```python
from build123d import *

# Parameters (mm, degrees)
F0_R     = 15
F0_R_2   = 9.5
F0_R_3   = 4.5
F0_R_4   = 2.55
F1_DEPTH = 15
F3_DEPTH = 3
F4_DEPTH = 10
F5_DEPTH = 5


with BuildPart() as f1:
    # F0 (on Top) → F1 (new body)
    with BuildSketch(Plane.XY):
        Circle(F0_R)
        Circle(F0_R_2, mode=Mode.SUBTRACT)
        Circle(F0_R_2)
        Circle(F0_R_3, mode=Mode.SUBTRACT)
        Circle(F0_R_3)
        Circle(F0_R_4, mode=Mode.SUBTRACT)
    extrude(amount=F1_DEPTH)

    # F2 (on face) → F3 (cut)
    with BuildSketch(Plane.XY.offset(15)):
        Polygon((2.4248711306, -4.2), (4.8497422612, 0), (2.4248711306, 4.2), (-2.4248711306, 4.2), (-4.8497422612, 0), (-2.4248711306, -4.2), align=None)
    extrude(amount=-F3_DEPTH, mode=Mode.SUBTRACT)

    # F0 (on Top) → F4 (cut)
    with BuildSketch(Plane.XY):
        Circle(F0_R_3)
        Circle(F0_R_4, mode=Mode.SUBTRACT)
    extrude(amount=F4_DEPTH, mode=Mode.SUBTRACT)

    # F0 (on Top) → F5 (join)
    with BuildSketch(Plane.XY):
        Circle(F0_R)
        Circle(F0_R_2, mode=Mode.SUBTRACT)
    extrude(amount=-F5_DEPTH)


solid = f1.part
```
Input: part model. Units: mm. Frame: model coordinates. A direction names the side the tool comes from. Give positions to 0.01 mm unless a question says otherwise; leave off trailing zeros. Order: outer loops, then holes, each group sorted by start corner. A loop starts at its lowest first (then second) coordinate and runs counter-clockwise, first axis right, second up. Notation, with made-up numbers: M -34,82.5 L -6,82.5 A29 cw -6,120.5 Z; hole C 87,-21 d8. An arc over 180 degrees is marked long. Return JSON: item names as keys, results as strings.
1) Section query A-A on x = 0. Output: boundary loops of the cut face in (y, z).
Taken from the geometry:
{"outline": "M -15,-5 L -9.5,-5 L -9.5,0 L -4.5,0 L -4.5,10 L -2.55,10 L -2.55,12 L -4.2,12 L -4.2,15 L -15,15 Z; M 2.55,10 L 4.5,10 L 4.5,0 L 9.5,0 L 9.5,-5 L 15,-5 L 15,15 L 4.2,15 L 4.2,12 L 2.55,12 Z"}
2) Section query B-B on z = 9. Output: boundary loops of the cut face in (x, y).
Taken from the geometry:
{"outline": "C 0,0 d30; hole C 0,0 d9"}
3) Line query: L1, parallel to Y at x = 0, z = 5.5; L2, parallel to Z at x = 6, y = -6; L3, parallel to X at y = -1.5, z = 2.25. Output: solid intervals per line, ascending. Write a range as [from, to].
Taken from the geometry:
{"L1": "y = [-15, -4.5], [4.5, 15]", "L2": "z = [0, 15]", "L3": "x = [-14.92, -4.24], [4.24, 14.92]"}
4) Mould query, pull axis Y, two halves, no side actions, for faces 4 (the face through (3, 4, 15)), 5 (the face through (0, -4.2, 14)), 6 (the face through (-14.985, 0.66, 5.14)). Classes: released by +Y, released by -Y, zero draft, split by the parting line, or undercut.
Taken from the geometry:
{"face 4": "zero draft", "face 5": "undercut", "face 6": "split by the parting line"}
5) Access query for faces 1 (the face through (-3.654, -2.071, 13.521)), 2 (the face through (-0.59, 4.46, 4.93)), 3 (the face through (0, -10, -5)). Directions: +Z, -Z, +X, -X, +Y, -Y. A direction counts if a zero-diameter tool reaches every point of the face in a straight line with its end or side. Return the directions, or none.
Taken from the geometry:
{"face 1": "+Z", "face 2": "-Z", "face 3": "-Z, +X, -X, +Y, -Y"}
6) Contact query for flat-ended pins moving along their axis: pin 1 (3.5 mm diameter, centred on x = -1, z = 13, fed in from -Y); pin 2 (1.5 mm diameter, centred on x = 10.5, z = 0, fed in from -Y); pin 3 (8 mm diameter, centred on x = -9.5, z = 5.5, fed in from -Y); pin 4 (1.5 mm diameter, centred on y = -11.5, z = -2.5, fed in from -X). Output: stop coordinate, or through.
Taken from the geometry:
{"pin 1": "stops at y = -15", "pin 2": "stops at y = -11.4", "pin 3": "stops at y = -13.96", "pin 4": "stops at x = -10.46"}
7) Section query D-D on x = -9. Output: boundary loops of the cut face in (y, z), and give its area (3 significant figures).
Taken from the geometry:
{"outline": "M -12,-5 L -3.04,-5 L -3.04,0 L 3.04,0 L 3.04,-5 L 12,-5 L 12,15 L -12,15 Z", "area": "450 mm2"}
8) Section query C-C on y = 0.5. Output: boundary loops of the cut face in (x, z).
Taken from the geometry:
{"outline": "M -14.99,-5 L -9.49,-5 L -9.49,0 L -4.47,0 L -4.47,10 L -2.5,10 L -2.5,12 L -4.56,12 L -4.56,15 L -14.99,15 Z; M 2.5,10 L 4.47,10 L 4.47,0 L 9.49,0 L 9.49,-5 L 14.99,-5 L 14.99,15 L 4.56,15 L 4.56,12 L 2.5,12 Z"}
